Part model, mm, in its own coordinate system. A direction names the side the tool comes from. Coordinates: 2 decimals unless noted, no trailing zeros. Order: outer loops, then holes, each group sorted by start corner. A loop starts at its lowest first (then second) coordinate and runs counter-clockwise, first axis right, second up.
Autodesk Inventor part; units mm, degrees
ref_plane "YZ Plane" through (0, 0, 0) normal (1, 0, 0) x (0, 1, 0)
ref_plane "XZ Plane" through (0, 0, 0) normal (0, 1, 0) x (-1, 0, 0)
ref_plane "XY Plane" through (0, 0, 0) normal (0, 0, 1) x (1, 0, 0)
sketch "Szkic1" plane through (0, 0, 0) normal (0, 0, 1) x (1, 0, 0)
  line L0 (-2.2485, 0) -> (12.0414, 0)
  line L1 (0, -4.2485) -> (0, 24.0414)
  line L2 (10, 0) -> (1, 0)
  line L3 (0, 1) -> (0, 20)
  line L4 (2, 20) -> (2, 3)
  line L5 (3, 2) -> (10, 2)
  line L6 (0, 20) -> (2, 20)
  line L7 (10, 0) -> (10, 2)
  arc A0 (2, 3) -> (3, 2) centre (3, 3) ccw
  arc A1 (0, 1) -> (1, 0) centre (1, 1) ccw
  point P0 (0, 0)
  dimension "d0" = 20
  dimension "d1" = 10
  dimension "d2" = 2
  dimension "d3" = 1
extrude "Wyciągnięcie proste1" add sketch "Szkic1" along normal blind 86 contours A1 L1 L6 L4 A0 L5 L7 L0
properties part number "kątownik_mały3" material "Aluminium 6061"
(1) Slice it at A-A, the plane z = 74. Give the cut face in (x, y).
(2) Slice it at B-B, the plane x = 4. Give the cut face in (y, z).
(3) Tool access for faces 1 (the face through (10, 1, 42)), 2 (the face through (2, 12, 42)): list every direction of +Z, -Z, +X, -X, +Y, -Y with a clear straight run to the whole face (end or side of a thin tool).
(4) Probe line 1 (Y direction, x = 4.25, z = 52.5); line 2 (Y direction, x = 2.25, z = 69.5). List the from-to ranges inside material, lowest first.
(5) Drop flat-ended pins along their axis: pin 1 (3.5 mm diameter, centred on x = 6.5, z = 31.5, fed in from +Y); pin 2 (1.5 mm diameter, centred on x = 4.5, y = 10.5, fed in from -Z); pin 3 (5 mm diameter, centred on y = 15.5, z = 39, fed in from +X). Give the stop position or say it passes through.
Here are the results:
1. outline: (0, 1) arc R1 ccw to (1, 0) - (10, 0) - (10, 2) - (3, 2) arc R1 cw to (2, 3) - (2, 20) - (0, 20) - close
2. outline: (0, 0) - (2, 0) - (2, 86) - (0, 86) - close
3. face 1: +Z, -Z, +X, +Y, -Y
3. face 2: +Z, -Z, +X, +Y
4. line 1: y = 0 to 2
4. line 2: y = 0 to 2.34
5. pin 1: stops at y = 2
5. pin 2: passes through
5. pin 3: stops at x = 2
